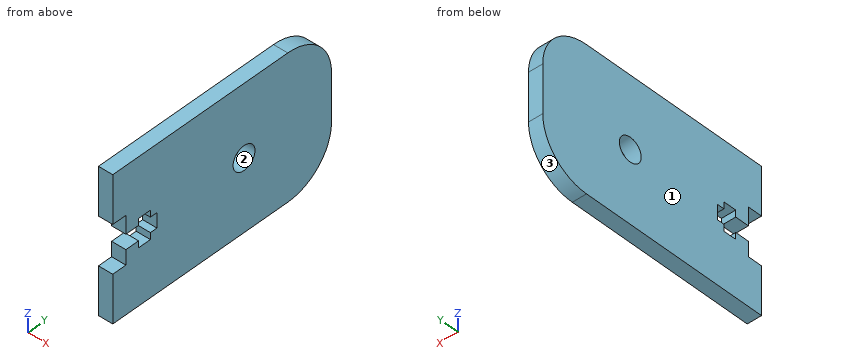
```python
from build123d import *

# Parameters (mm, degrees)
SKETCH1_W                 = 30
SKETCH1_H                 = 50
BOSS_EXTRUDE1_DEPTH       = 3
FILLET1_R                 = 10
SKETCH2_W                 = 10
SKETCH2_H                 = 3
CUT_EXTRUDE1_DEPTH        = 3
F_5_0MM_DOWEL_HOLE1_D     = 5
F_5_0MM_DOWEL_HOLE1_DEPTH = 3
F_5_0MM_DOWEL_HOLE1_TIP   = 1.502151548
CUT_EXTRUDE2_DEPTH        = 3


with BuildPart() as part:
    # Sketch1 → Boss-Extrude1 (new body)
    with BuildSketch(Plane(origin=(0, 0, 0), x_dir=(0, 0, -1), z_dir=(1, 0, 0))):
        with Locations((15, 25)):
            Rectangle(SKETCH1_W, SKETCH1_H)
    extrude(amount=BOSS_EXTRUDE1_DEPTH)

    # Fillet1
    fillet1_edges = [part.edges().sort_by_distance(p)[0] for p in [
        (1.5, 50, 0),
        (1.5, 50, -30),
    ]]
    fillet(fillet1_edges, radius=FILLET1_R)

    # Sketch2 → Cut-Extrude1 (cut)
    with BuildSketch(Plane(origin=(3, 0, 0), x_dir=(0, 0, -1), z_dir=(1, 0, 0))):
        with Locations((15, 1.5)):
            Rectangle(SKETCH2_W, SKETCH2_H)
    extrude(amount=-CUT_EXTRUDE1_DEPTH, mode=Mode.SUBTRACT)

    # Ø5.0mm Dowel Hole1
    with Locations(Plane(origin=(3, 0, 0), x_dir=(0, 0, -1), z_dir=(1, 0, 0))):
        with Locations((15, 30)):
            Hole(F_5_0MM_DOWEL_HOLE1_D / 2, depth=F_5_0MM_DOWEL_HOLE1_DEPTH)
            with Locations((0, 0, -(F_5_0MM_DOWEL_HOLE1_DEPTH + F_5_0MM_DOWEL_HOLE1_TIP / 2))):  # 118° drill point
                Cone(0, F_5_0MM_DOWEL_HOLE1_D / 2, F_5_0MM_DOWEL_HOLE1_TIP, mode=Mode.SUBTRACT)

    # Sketch5 → Cut-Extrude2 (cut)
    with BuildSketch(Plane(origin=(3, 0, 0), x_dir=(0, 0, -1), z_dir=(1, 0, 0))):
        Polygon((13.796178669, 3), (13.796178669, 5.9), (12.396178669, 5.9), (12.396178669, 8.6), (13.796178669, 8.6), (13.796178669, 10.1), (16.896178669, 10.1), (16.896178669, 8.6), (18.296178669, 8.6), (18.296178669, 5.9), (16.896178669, 5.9), (16.896178669, 3), align=None)
    extrude(amount=-CUT_EXTRUDE2_DEPTH, mode=Mode.SUBTRACT)


solid = part.part
```
Verification items for the finished model (mm, model axes). Face numbers are marked on the shaded views. Coordinates: 2 decimals unless noted, no trailing zeros. Loops run counter-clockwise (first coordinate to the right, second up) from the corner with the lowest first, then second, coordinate; pieces in that order, holes last. Notation, with made-up numbers: (59, -23.75) - (92, -23.75) arc R24 ccw to (92, -11.75) - close; hole circle Ø2 at (47, 73). An arc over 180 degrees is marked (long way). Answer as a JSON object with one key per item and string values.
(1) Go/stop test with flat-tipped pins: pin 1 Ø1.5 at (x, z) = (2, -13.5) entering from -Y; pin 2 Ø1.5 at (x, z) = (2.5, -24) entering from +Y; pin 3 Ø0.9 at (x, z) = (2, -15) entering from -Y. Record where each tip stops, or that it passes through.
Response:
{"pin 1": "stops at y = 3", "pin 2": "stops at y = 49.46", "pin 3": "stops at y = 10.1"}
(2) Cross-section at C-C, the plane x = 1.05. Record the boundary of the cut face in (y, z).
Response:
{"outline": "(0, -30) - (40, -30) arc R10 ccw to (50, -20) - (50, -10) arc R10 ccw to (40, 0) - (0, 0) - (0, -10) - (3, -10) - (3, -13.8) - (5.9, -13.8) - (5.9, -12.4) - (8.6, -12.4) - (8.6, -13.8) - (10.1, -13.8) - (10.1, -16.9) - (8.6, -16.9) - (8.6, -18.3) - (5.9, -18.3) - (5.9, -16.9) - (3, -16.9) - (3, -20) - (0, -20) - close; hole circle Ø5 at (30, -15)"}
(3) Mould release check, pull along Y, two halves, no side actions. Record for the marked faces 1, 2 and 3: pulls with the +Y half, pulls with the -Y half, needs draft (parallel to the pull), parting line crosses it, or undercut.
Response:
{"face 1": "needs draft", "face 2": "undercut", "face 3": "pulls with the +Y half"}
(4) Scan lines: line 1 along Z through (x, y) = (1.3, 30); line 2 along Y through (x, z) = (1.55, -15); line 3 along Y through (x, z) = (2.9, -18.25). Record each from-to range of solid material in increasing order.
Response:
{"line 1": "z = -30 to -17.5, -12.5 to 0", "line 2": "y = 10.1 to 27.5, 32.5 to 50", "line 3": "y = 3 to 5.9, 8.6 to 50"}
(5) Cross-section at D-D, the plane z = -2. Record the boundary of the cut face in (x, y).
Response:
{"outline": "(0, 0) - (3, 0) - (3, 46) - (0, 46) - close"}
(6) Cross-section at A-A, the plane z = -15. Record the boundary of the cut face in (x, y).
Response:
{"outline": "(0, 10.1) - (3, 10.1) - (3, 27.5) - (0, 27.5) - close; (0, 32.5) - (3, 32.5) - (3, 50) - (0, 50) - close"}
(7) Cross-section at B-B, the plane y = 30. Record the boundary of the cut face in (x, z), then the cut area to 3 significant figures.
Response:
{"outline": "(0, -30) - (3, -30) - (3, -17.5) - (0, -17.5) - close; (0, -12.5) - (3, -12.5) - (3, 0) - (0, 0) - close", "area": "75.0 mm²"}
